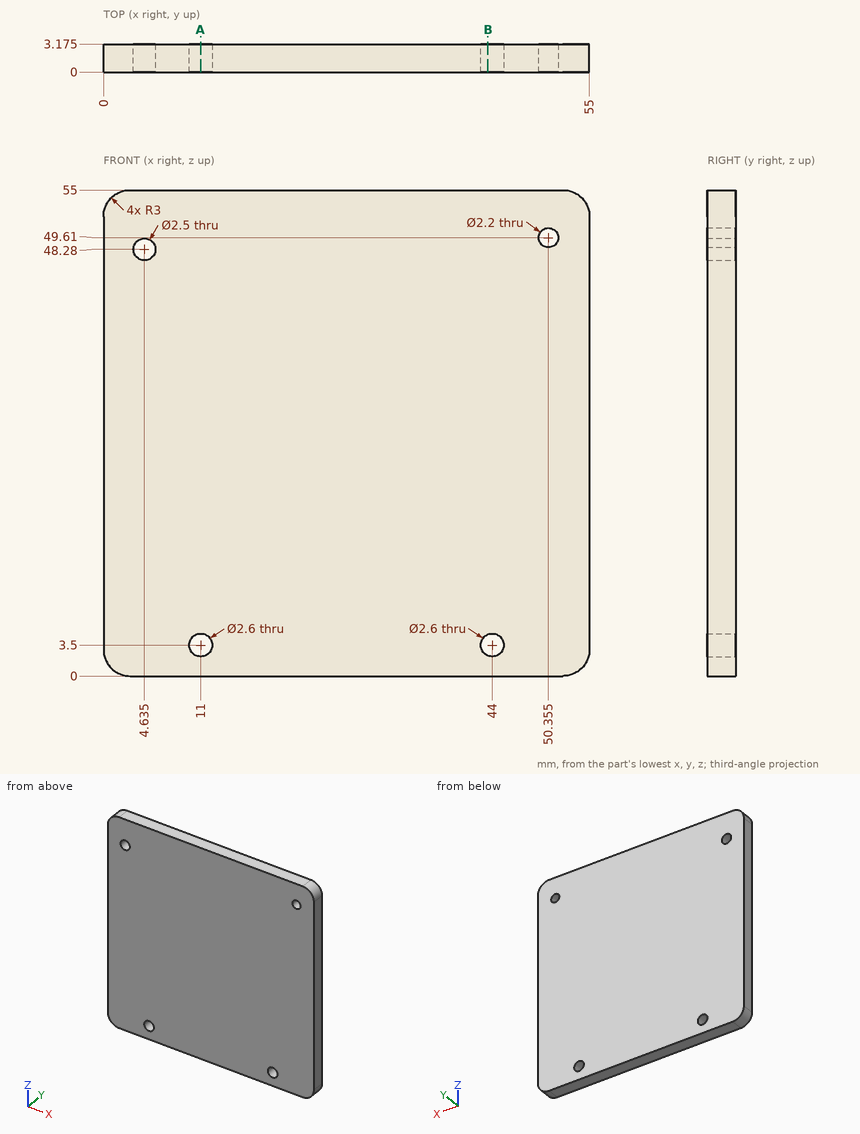
Geometry: see drawing. Coordinates: mm, zero at the bounding-box minimum. Round coordinates to 2 decimals unless told otherwise and drop trailing zeros. Loops run counter-clockwise (first coordinate to the right, second up) from the corner with the lowest first, then second, coordinate; pieces in that order, holes last. Notation, with made-up numbers: M 87,16 L 145,16 A19 ccw 145,20 Z; hole C 2.5,38 d3. An arc over 180 degrees is marked long. Use a Markdown table: item, result. Add a question column.
1. Ray query, line 1 along Z through (x, y) = (11, 2.1); line 2 along X through (y, z) = (1.05, 3.5); line 3 along X through (y, z) = (1.85, 49.61) (3 decimals). Return the intervals inside material, ascending. Write a range as [from, to].
2. Cut plane A-A, the plane x = 11. Output: boundary loops of the cut face in (y, z) (3 decimals), and give its area (3 significant figures).
3. Cut plane B-B, the plane x = 43.5. Output: boundary loops of the cut face in (y, z) (3 decimals), and give its area (3 significant figures).
Solution:
| question | item | result |
|---|---|---|
| 1 | line 1 | z = [0, 2.2], [4.8, 55] |
| 1 | line 2 | x = [0, 9.7], [12.3, 42.7], [45.3, 55] |
| 1 | line 3 | x = [0, 49.255], [51.455, 55] |
| 2 | outline | M 0,0 L 3.175,0 L 3.175,2.2 L 0,2.2 Z; M 0,4.8 L 3.175,4.8 L 3.175,55 L 0,55 Z |
| 2 | area | 166 mm2 |
| 3 | outline | M 0,0 L 3.175,0 L 3.175,2.3 L 0,2.3 Z; M 0,4.7 L 3.175,4.7 L 3.175,55 L 0,55 Z |
| 3 | area | 167 mm2 |
